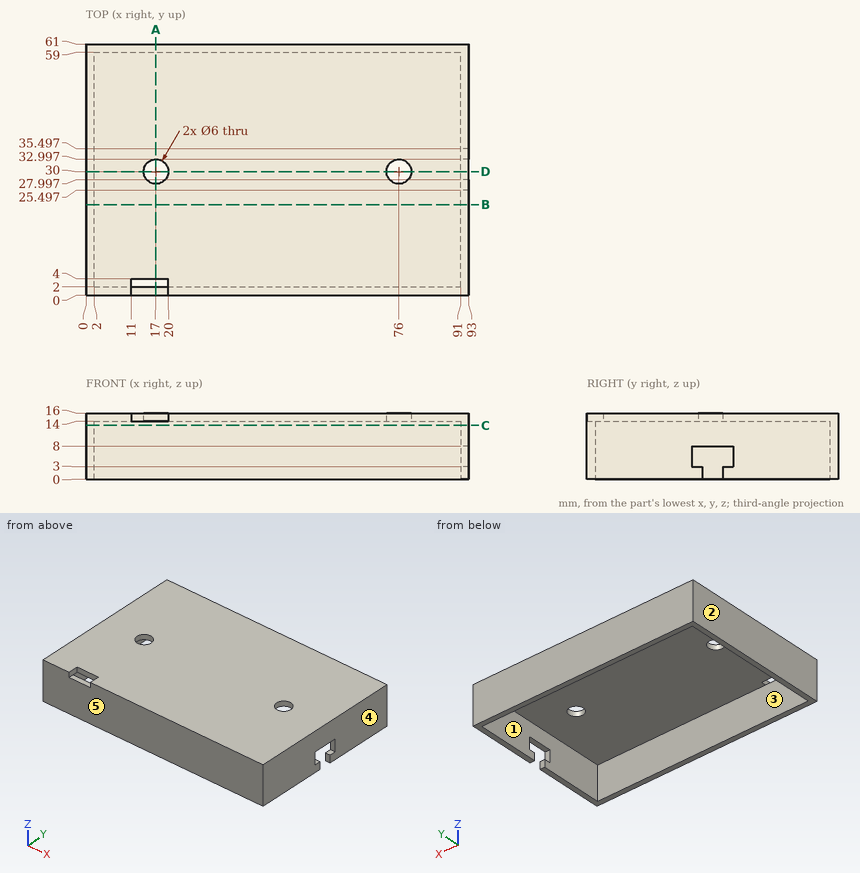
Geometry: see drawing. Coordinates: mm, zero at the bounding-box minimum. A direction names the side the tool comes from. Round coordinates to 2 decimals unless told otherwise and drop trailing zeros. Loops run counter-clockwise (first coordinate to the right, second up) from the corner with the lowest first, then second, coordinate; pieces in that order, holes last. Notation, with made-up numbers: M -2,25.5 L 34,25.5 A12 cw 34,38.5 Z; hole C -29.75,34.5 d7. An arc over 180 degrees is marked long. Use a Markdown table: item, result. Add a question column.
1. Section query C-C on z = 13. Return the cut outline in (x, y), then the cut area to 3 significant figures.
2. Section query A-A on x = 17. Return the cut outline in (y, z).
3. Contact query for flat-ended pins moving along their axis: P1, Ø0.6, axis at x = 92, y = 32, coming from the -Z side; P2, Ø1, axis at x = 36, y = 32, coming from the -Z side. Output: stop coordinate, or through.
4. Reachability of the marked faces 1 and 2 from +Z, -Z, +X, -X, +Y, -Y: full face, straight path, thin tool, end or side. Return the list, or none.
5. Section query D-D on y = 30. Return the cut outline in (x, z), then the cut area to 3 significant figures.
6. Line query: line 1 (Y direction, x = 76, z = 14.75); line 2 (X direction, y = 37.5, z = 7.5); line 3 (Y direction, x = 56.5, z = 4.75). Output: solid intervals per line, ascending.
7. Section query B-B on y = 22. Return the cut outline in (x, z), then the cut area to 3 significant figures.
8. Mould query, pull axis Y, two halves, no side actions, for the marked faces 3, 4 and 5. Classes: pulls with the +Y half, pulls with the -Y half, needs draft (parallel to the pull), parting line crosses it, or undercut.
Reported:
| question | item | result |
|---|---|---|
| 1 | outline | M 0,0 L 93,0 L 93,61 L 0,61 Z; hole M 2,2 L 91,2 L 91,59 L 2,59 Z |
| 1 | area | 600 mm² |
| 2 | outline | M 0,0 L 2,0 L 2,14 L 0,14 Z; M 4,14 L 27,14 L 27,16 L 4,16 Z; M 33,14 L 59,14 L 59,0 L 61,0 L 61,16 L 33,16 Z |
| 3 | P1 | stops at z = 8 |
| 3 | P2 | stops at z = 14 |
| 4 | face 1 | -Z |
| 4 | face 2 | +Z, -Z, -X, +Y, -Y |
| 5 | outline | M 0,0 L 2,0 L 2,14 L 14,14 L 14,16 L 0,16 Z; M 20,14 L 73,14 L 73,16 L 20,16 Z; M 79,14 L 91,14 L 91,8 L 93,8 L 93,16 L 79,16 Z |
| 5 | area | 202 mm² |
| 6 | line 1 | y = 0 to 27, 33 to 61 |
| 6 | line 2 | x = 0 to 2, 91 to 93 |
| 6 | line 3 | y = 0 to 2, 59 to 61 |
| 7 | outline | M 0,0 L 2,0 L 2,14 L 91,14 L 91,0 L 93,0 L 93,16 L 0,16 Z |
| 7 | area | 242 mm² |
| 8 | face 3 | undercut |
| 8 | face 4 | needs draft |
| 8 | face 5 | pulls with the -Y half |
